Part print with two shaded views. Sizes in mm from the minimum x, y, z corner. A direction names the side the tool comes from. Round coordinates to 2 decimals unless told otherwise and drop trailing zeros. Loops run counter-clockwise (first coordinate to the right, second up) from the corner with the lowest first, then second, coordinate; pieces in that order, holes last.
(1) Flat gauge pins, fed straight in: pin 1 (5 mm diameter, centred on x = 17, y = 4.5, fed in from -Z); pin 2 (5 mm diameter, centred on x = 26.5, y = 1, fed in from -Z); pin 3 (4 mm diameter, centred on x = 7.5, z = 4, fed in from -Y). Where does each tip first touch, or does it go through?
(2) Cut at B-B on z = 4.25. List the corners of the cut face in (x, y).
(3) Cut at C-C on x = 7. List the corners of the cut face in (y, z), then the cut area to 3 significant figures.
(4) Cut at D-D on x = 2.25. List the corners of the cut face in (y, z), then the cut area to 3 significant figures.
(5) Tool access for the marked faces 1 and 2: list every direction of +Z, -Z, +X, -X, +Y, -Y with a clear straight run to the whole face (end or side of a thin tool).
(6) Cut at A-A on y = 4.25. List the corners of the cut face in (x, z), then the cut area to 4 significant figures.
(7) Mould opens along Y. For the marked faces 3, 4 and 5 say: +Y half, -Y half, draft (parallel to the pull), parting line (faces both ways), or undercut.
(8) Probe probe 1 along Y at (x, z) = (19, 4.25); probe 2 along Y at (x, z) = (13.75, 2.5). List the from-to ranges inside material, lowest first.
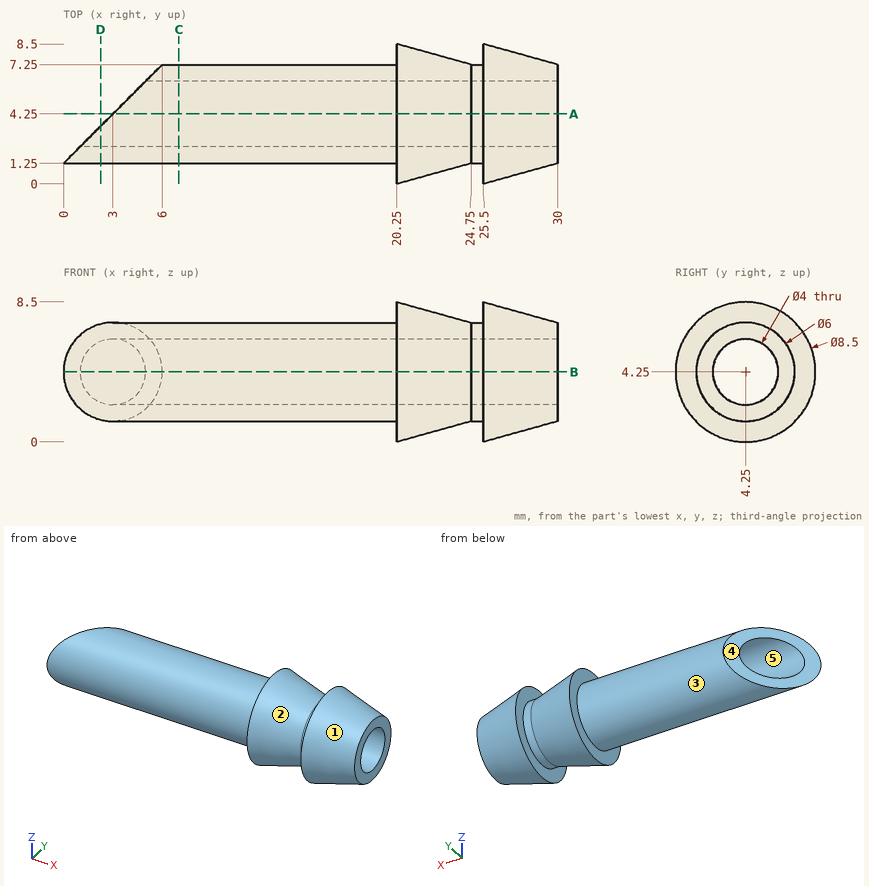
Final values:
1. pin 1: stops at z = 1.25
1. pin 2: stops at z = 0.11
1. pin 3: stops at y = 1.25
2. outline: (0, 1.25) - (20.25, 1.25) - (20.25, 0) - (24.75, 1.25) - (25.5, 1.25) - (25.5, 0) - (30, 1.25) - (30, 2.25) - (1, 2.25) - close; (5, 6.25) - (30, 6.25) - (30, 7.25) - (25.5, 8.5) - (25.5, 7.25) - (24.75, 7.25) - (20.25, 8.5) - (20.25, 7.25) - (6, 7.25) - close
3. outline: circle Ø6 at (4.25, 4.25); hole circle Ø4 at (4.25, 4.25)
3. area: 15.7 mm2
4. outline: (3.5, 1.35) - (3.5, 2.4) arc R2 cw to (3.5, 6.1) - (3.5, 7.15) arc R3 ccw to start
4. area: 6.33 mm2
5. face 1: +X
5. face 2: none
6. outline: (3, 1.25) - (20.25, 1.25) - (20.25, 0) - (24.75, 1.25) - (25.5, 1.25) - (25.5, 0) - (30, 1.25) - (30, 2.25) - (3, 2.25) - close; (3, 6.25) - (30, 6.25) - (30, 7.25) - (25.5, 8.5) - (25.5, 7.25) - (24.75, 7.25) - (20.25, 8.5) - (20.25, 7.25) - (3, 7.25) - close
6. area: 65.25 mm2
7. face 3: parting line
7. face 4: +Y half
7. face 5: undercut
8. probe 1: y = 1.25 to 2.25, 6.25 to 7.25
8. probe 2: y = 1.81 to 3.28, 5.22 to 6.69
